Autodesk Inventor part; units mm, degrees
ref_plane "YZ Plane" through (0, 0, 0) normal (1, 0, 0) x (0, 1, 0)
ref_plane "XZ Plane" through (0, 0, 0) normal (0, 1, 0) x (-1, 0, 0)
ref_plane "XY Plane" through (0, 0, 0) normal (0, 0, 1) x (1, 0, 0)
ref_plane "Work Plane1" through (0, 42.0672, 0) normal (0, 0, 1) x (1, 0, 0)
sketch "Sketch1" plane through (0, 42.0672, 0) normal (0, 0, 1) x (1, 0, 0)
  line L0 (0, -42.0672) -> (482.346, -42.0672)
  line L1 (482.346, -42.0672) -> (482.346, -67.4672)
  line L2 (482.346, -67.4672) -> (0, -67.4672)
  line L3 (0, -67.4672) -> (0, -42.0672)
  line L4 (0, -67.4672) -> (0, -61.1172)
  line L5 (0, -61.1172) -> (482.346, -61.1172)
  line L6 (482.346, -61.1172) -> (482.346, -86.5172)
  line L7 (482.346, -86.5172) -> (0, -86.5172)
  line L8 (0, -86.5172) -> (0, -61.1172)
  dimension "d0" = 482.346
  dimension "d1" = 25.4
  dimension "d2" = 6.35
  dimension "d3" = 482.346
  dimension "d4" = 25.4
extrude "Extrusion1" add sketch "Sketch1" along normal blind 0.254 contours L5 L1 L2 L3 | L2 L6 L7 L8
sketch "Sketch2" plane through (0, -44.45, 0) normal (-1, 0, 0) x (0, 0, 1)
  line L0 (0, 25.4) -> (0, 0)
  line L1 (0, 0) -> (0.254, 0)
  line L2 (0.254, 25.4) -> (0.254, 0)
  line L3 (0, 25.4) -> (0.254, 25.4)
  point P0 (0, 44.45)
extrude "Extrusion2" add sketch "Sketch2" along normal blind 0.254
sketch "Sketch3" plane through (482.346, -44.45, 0) normal (1, 0, 0) x (0, 0, -1)
  line L0 (0, 0) -> (0, 25.4)
  line L1 (0, 25.4) -> (-0.254, 25.4)
  line L2 (-0.254, 0) -> (-0.254, 25.4)
  line L3 (0, 0) -> (-0.254, 0)
  point P0 (0, 44.45)
extrude "Extrusion3" add sketch "Sketch3" along normal blind 0.254
sketch "Sketch4" plane through (0, 42.0672, 0) normal (0, 0, -1) x (-1, 0, 0)
  line L0 (-482.6, -61.1172) -> (-482.346, -61.1172)
  line L1 (-482.346, -61.1172) -> (-482.346, -86.5172)
  line L2 (-482.346, -86.5172) -> (-482.6, -86.5172)
  line L3 (-482.6, -86.5172) -> (-482.6, -61.1172)
  line L4 (0.254, -61.1172) -> (0, -61.1172)
  line L5 (0, -61.1172) -> (0, -86.5172)
  line L6 (0, -86.5172) -> (0.254, -86.5172)
  line L7 (0.254, -86.5172) -> (0.254, -61.1172)
  point P0 (0, -42.0672)
  dimension "d11" = 0.254
  dimension "d12" = 25.4
  dimension "d13" = 0.254
  dimension "d14" = 25.4
extrude "Extrusion4" add sketch "Sketch4" along normal blind 25.4
properties part number "Cloth"
Verification items for the finished model (mm, model axes). A direction names the side the tool comes from. Coordinates: 2 decimals unless noted, no trailing zeros. Write each loop counter-clockwise with the first axis right and the second up, starting at its lowest first coordinate (ties: lowest second). Pieces come first, ordered by that corner, then holes. Notation, with made-up numbers: M -18,64.25 L 12,64.25 A17 ccw 12,81.25 Z; hole C 23,-21 d1. An arc over 180 degrees is marked long. Answer as a JSON object with one key per item and string values. Group by question number.
(1) Cross-section at B-B, the plane y = -28.5. Record the cut outline in (x, z), and give its area (3 significant figures).
(2) Material ranges on line 1 (X direction, y = -38, z = -17); line 2 (Z direction, x = 239, y = -36.75), recorded low to high.
(3) Cross-section at A-A, the plane z = -11.75. Record the cut outline in (x, y).
(4) Release check for a two-part mould opening along X. For faces 1 (the face through (-0.254, -32, -13)), 2 (the face through (482.6, -32, -12)), 3 (the face through (0, -32, -13)) record: +X half, -X half, draft (parallel to the pull), parting line (faces both ways), or undercut.
(5) Tool access check on faces 4 (the face through (238, -32, 0)), 5 (the face through (238, -32, 0.254)). Record the directions out of +Z, -Z, +X, -X, +Y, -Y that give a thin tool (end or side, any length) a straight path to the whole face; none if there is none.
(6) Cross-section at C-C, the plane x = 377. Record the cut outline in (y, z).
(7) Gauge pin test, flat end, axial feed: pin 1 (1.5 mm diameter, centred on x = 308, y = -36, fed in from -Z). Record the tip position at first contact, or that the pin passes through.
Reply:
{
 "1": {"outline": "M -0.25,-25.4 L 0,-25.4 L 0,0 L 482.35,0 L 482.35,-25.4 L 482.6,-25.4 L 482.6,0.25 L -0.25,0.25 Z", "area": "136 mm²"},
 "2": {"line 1": "-0.25 to 0, 482.35 to 482.6", "line 2": "0 to 0.25"},
 "3": {"outline": "M -0.25,-44.45 L 0,-44.45 L 0,-19.05 L -0.25,-19.05 Z; M 482.35,-44.45 L 482.6,-44.45 L 482.6,-19.05 L 482.35,-19.05 Z"},
 "4": {"face 1": "-X half", "face 2": "+X half", "face 3": "undercut"},
 "5": {"face 4": "-Z, +Y, -Y", "face 5": "+Z, +X, -X, +Y, -Y"},
 "6": {"outline": "M -44.45,0 L -19.05,0 L -19.05,0.25 L -44.45,0.25 Z"},
 "7": {"pin 1": "z = 0"}
}
